```python
from build123d import *

# Parameters (mm, degrees)
ESQUISSE1_R             = 4.1
BOSS_EXTRU_1_DEPTH      = 5
ENL_V_MAT_EXTRU_1_DEPTH = 13.628539086
D_POUILLE1_ANGLE        = 19.963654133


with BuildPart() as part:
    # Esquisse1 → Boss.-Extru.1 (new body)
    with BuildSketch(Plane(origin=(0, 0, 0), x_dir=(-1, 0, 0), z_dir=(0, 0, -1))):
        with Locations((-4.099999911, 4.100000055)):
            Circle(ESQUISSE1_R)
    extrude(amount=-BOSS_EXTRU_1_DEPTH)

    # Esquisse2 → Enlèv. mat.-Extru.1 (cut, through all)
    with BuildSketch(Plane.XY.offset(5)):
        Polygon((7.076344, 4.476), (7.005749, 4.846069), (6.889329, 5.204373), (6.72892, 5.545261), (6.527051, 5.863356), (6.286906, 6.153641), (6.012272, 6.41154), (5.70748, 6.632984), (5.377338, 6.814481), (5.027051, 6.95317), (4.662144, 7.046862), (4.288372, 7.09408), (3.911628, 7.09408), (3.537856, 7.046862), (3.172949, 6.95317), (2.822662, 6.814481), (2.49252, 6.632984), (2.187728, 6.41154), (1.913094, 6.153641), (1.672949, 5.863356), (1.47108, 5.545261), (1.31067, 5.204373), (1.194251, 4.846069), (1.123656, 4.476), (1.1, 4.1), (1.123656, 3.724), (1.194251, 3.35393), (1.31067, 2.995626), (1.47108, 2.654739), (1.672949, 2.336644), (1.913094, 2.046359), (2.187728, 1.78846), (2.49252, 1.567016), (2.822662, 1.385519), (3.172949, 1.24683), (3.537856, 1.153138), (3.911628, 1.10592), (4.288372, 1.10592), (4.662144, 1.153138), (5.027051, 1.24683), (5.377338, 1.385519), (5.70748, 1.567016), (6.012272, 1.78846), (6.286906, 2.046359), (6.527051, 2.336644), (6.72892, 2.654739), (6.889329, 2.995626), (7.005749, 3.35393), (7.076344, 3.724), (7.1, 4.1), align=None)
    extrude(amount=-ENL_V_MAT_EXTRU_1_DEPTH, mode=Mode.SUBTRACT)

    # Dépouille1
    d_pouille1_faces = [part.faces().sort_by_distance(p)[0] for p in [
        (7.0410465, 4.6610345, 2.5),
        (6.947539, 5.025221, 2.5),
        (6.8091245, 5.374817, 2.5),
        (6.6279855, 5.7043085, 2.5),
        (6.4069785, 6.0084985, 2.5),
        (6.149589, 6.2825905, 2.5),
        (5.859876, 6.522262, 2.5),
        (5.542409, 6.7237325, 2.5),
        (5.2021945, 6.8838255, 2.5),
        (4.8445975, 7.000016, 2.5),
        (4.475258, 7.070471, 2.5),
        (4.1, 7.09408, 2.5),
        (3.724742, 7.070471, 2.5),
        (3.3554025, 7.000016, 2.5),
        (2.9978055, 6.8838255, 2.5),
        (2.657591, 6.7237325, 2.5),
        (2.340124, 6.522262, 2.5),
        (2.050411, 6.2825905, 2.5),
        (1.7930215, 6.0084985, 2.5),
        (1.5720145, 5.7043085, 2.5),
        (1.390875, 5.374817, 2.5),
        (1.2524605, 5.025221, 2.5),
        (1.1589535, 4.6610345, 2.5),
        (1.111828, 4.288, 2.5),
        (1.111828, 3.912, 2.5),
        (1.1589535, 3.538965, 2.5),
        (1.2524605, 3.174778, 2.5),
        (1.390875, 2.8251825, 2.5),
        (1.5720145, 2.4956915, 2.5),
        (1.7930215, 2.1915015, 2.5),
        (2.050411, 1.9174095, 2.5),
        (2.340124, 1.677738, 2.5),
        (2.657591, 1.4762675, 2.5),
        (2.9978055, 1.3161745, 2.5),
        (3.3554025, 1.199984, 2.5),
        (3.724742, 1.129529, 2.5),
        (4.1, 1.10592, 2.5),
        (4.475258, 1.129529, 2.5),
        (4.8445975, 1.199984, 2.5),
        (5.2021945, 1.3161745, 2.5),
        (5.542409, 1.4762675, 2.5),
        (5.859876, 1.677738, 2.5),
        (6.149589, 1.9174095, 2.5),
        (6.4069785, 2.1915015, 2.5),
        (6.6279855, 2.4956915, 2.5),
        (6.8091245, 2.8251825, 2.5),
        (6.947539, 3.174778, 2.5),
        (7.0410465, 3.538965, 2.5),
        (7.088172, 3.912, 2.5),
        (7.088172, 4.288, 2.5),
    ]]
    draft(d_pouille1_faces, Plane(origin=(4.099999911, 4.100000055, 5), x_dir=(1, 0, 0), z_dir=(0, 0, 1)), D_POUILLE1_ANGLE)


solid = part.part
```
The listing builds one solid part. Answer for the finished solid, in the listing's coordinates (mm). Give positions to 0.01 mm unless a question says otherwise; leave off trailing zeros. Order: outer loops, then holes, each group sorted by start corner. A loop starts at its lowest first (then second) coordinate and runs counter-clockwise, first axis right, second up. Notation, with made-up numbers: (52.25, -38.5) - (90.25, -38.5) arc R11 cw to (90.25, -22.5) - close; hole circle Ø3 at (6, -14.5). An arc over 180 degrees is marked (long way). Answer in a Markdown table with one row per item. Add a question column.
Q1. Find the intervals of material crossed by line 1 along Y through (x, z) = (3.5, 1.1); line 2 along Y through (x, z) = (4.75, 4.05); line 3 along X through (y, z) = (4.75, 0.8), in increasing order. Write a range as [from, to].
Q2. The part is cut by section A-A (y = 2.5). Determine the outline of the cut face in (x, z).
Q3. Given P1, Ø1, axis at y = 4.5, z = 2, coming from the +X side; P2, Ø1.5, axis at x = 2.5, z = 3, coming from the -Y side, each flat-ended and moving along its own axis, determine where each tip first touches the part or whether it passes through.
Determined:
| question | item | result |
|---|---|---|
| 1 | line 1 | y = [0.04, 2.64], [5.56, 8.16] |
| 1 | line 2 | y = [0.05, 1.53], [6.67, 8.15] |
| 1 | line 3 | x = [0.05, 2.78], [5.42, 8.15] |
| 2 | outline | (0.33, 0) - (7.87, 0) - (7.87, 5) - (6.63, 5) - (6.3, 4.24) - (5.8, 3.18) - (5.42, 2.46) - (5.12, 1.96) - (4.85, 1.62) - (4.62, 1.38) - (4.41, 1.23) - (4.2, 1.16) - (4, 1.16) - (3.79, 1.23) - (3.58, 1.38) - (3.35, 1.62) - (3.08, 1.96) - (2.78, 2.46) - (2.4, 3.18) - (1.9, 4.24) - (1.57, 5) - (0.33, 5) - close |
| 3 | P1 | stops at x = 8.2 |
| 3 | P2 | stops at y = 0.09 |
